Design review of the part built by this model. Coordinates are the model's own, in mm. Face numbers are marked on the shaded views. A direction names the side the tool comes from. Coordinates: 2 decimals unless noted, no trailing zeros. Loops run counter-clockwise (first coordinate to the right, second up) from the corner with the lowest first, then second, coordinate; pieces in that order, holes last. Notation, with made-up numbers: (-34.75, 20.25) - (-18.75, 20.25) arc R25 ccw to (-18.75, 53.25) - close; hole circle Ø1 at (12.5, 20). An arc over 180 degrees is marked (long way). Use one line per item in the form item = value. Start each with the question number.
(1) The part is to be moulded in two halves that separate along X. For the marked faces 3, 4, 5 and 6, say which applies: pulls with the +X half, pulls with the -X half, needs draft (parallel to the pull), parting line crosses it, or undercut.
(2) Add section D-D (x = 55.7). State the section outline as (y, z) points.
(3) For L1, parallel to X at y = 6.5, z = -1.35; L2, parallel to Y at x = 55.7, z = -3.3; L3, parallel to X at y = 19.5, z = -1.5, list the stretches that pass through material, from the lowest coordinate up.
(4) Add section C-C (y = 9.25). State the section outline as (x, z) points, plus the area to 3 significant figures.
(5) Tool access review of the marked faces 1 and 2: name each direction out of +Z, -Z, +X, -X, +Y, -Y from which nothing blocks a thin tool from reaching the whole face with its end or side.
(6) Add section A-A (y = -2). State the section outline as (x, z) points, plus the area to 3 significant figures.
(7) Clearance check with flat-ended pins moving along their axes: pin 1 Ø7.5 at (x, z) = (41, -9.5) entering from +Y; pin 2 Ø1.6 at (x, y) = (37, -1) entering from -Z. State where each tip first meets the part, or that it passes through.
(8) Add section B-B (x = 5.3). State the section outline as (y, z) points, plus the area to 3 significant figures.
Autodesk Inventor part; units mm, degrees
ref_plane "YZ Plane" through (0, 0, 0) normal (1, 0, 0) x (0, 1, 0)
ref_plane "XZ Plane" through (0, 0, 0) normal (0, 1, 0) x (-1, 0, 0)
ref_plane "XY Plane" through (0, 0, 0) normal (0, 0, 1) x (1, 0, 0)
sketch "Esquisse1" plane through (0, 0, 0) normal (0, 1, 0) x (-1, 0, 0)
  line L0 (0, 0) -> (-61, 0)
  line L1 (-61, 0) -> (-61, -15)
  line L2 (-61, -15) -> (0, -15)
  line L3 (0, -15) -> (0, 0)
  dimension "d0" = 15
  dimension "d1" = 61
extrude "Extrusion1" add sketch "Esquisse1" along normal blind 2
sketch "Esquisse2" plane through (0, 2, 0) normal (0, 1, 0) x (1, 0, 0)
  line L0 (0, 15) -> (0, 0)
  line L1 (0, 0) -> (9.5, 0)
  line L2 (9.5, 0) -> (9.5, 4.3)
  line L3 (0, 6.2) -> (0, 0)
  line L4 (0, 15) -> (9.5, 15)
  line L5 (9.5, 15) -> (9.5, 8.8)
  line L6 (9.5, 8.8) -> (0, 8.8)
  line L7 (0, 8.8) -> (0, 15)
  line L8 (0, 0) -> (61, 0) construction
  line L9 (30.5, 0) -> (30.5, 15) construction
  line L10 (61, 15) -> (61, 0)
  line L11 (61, 0) -> (51.5, 0)
  line L12 (51.5, 0) -> (51.5, 4.3)
  line L13 (51.5, 4.3) -> (61, 6.2)
  line L14 (61, 6.2) -> (61, 0)
  line L15 (61, 15) -> (51.5, 15)
  line L16 (51.5, 15) -> (51.5, 8.8)
  line L17 (51.5, 8.8) -> (61, 8.8)
  line L18 (61, 8.8) -> (61, 15)
  line L19 (0, 6.2) -> (2.5, 6.2)
  line L20 (2.5, 6.2) -> (9.5, 4.3)
  dimension "d33" = 2.6
  dimension "d34" = 6.2
  dimension "d36" = 4.5
  dimension "d37" = 2.5
  dimension "d38" = 7
extrude "Extrusion2" add sketch "Esquisse2" along normal blind 20
sketch "Esquisse3" plane through (0, 0, 0) normal (0, 0, 1) x (1, 0, 0)
  circle A0 centre (55.7, 16.5) radius 2
  line L0 (51.5, 2) -> (51.5, 22)
  circle A1 centre (55.7, 6.5) radius 2
  line L1 (51.5, 22) -> (61, 22)
  line L2 (0, 0) -> (61, 0)
  line L3 (51.5, 2) -> (9.5, 2) construction
  line L4 (30.5, 0) -> (30.5, 2) construction
  line L5 (9.5, 2) -> (51.5, 2) construction
  circle A2 centre (5.3, 16.5) radius 2
  circle A3 centre (5.3, 6.5) radius 2
  dimension "d10" = 4
  dimension "d11" = 4.2
  dimension "d12" = 4.2
  dimension "d40" = 10
  dimension "d41" = 4.5
extrude "Extrusion3" cut sketch "Esquisse3" against normal blind 20
sketch "Esquisse4" plane through (0, 0, 0) normal (0, -1, 0) x (1, 0, 0)
  circle A0 centre (44, -7.5) radius 5.15
  circle A1 centre (44, -7.5) radius 3.15
  line L0 (61, -6.2) -> (61, -8.8) construction
  line L1 (0, -8.8) -> (0, -6.2) construction
  line L2 (0, -15) -> (0, 0) construction
  line L3 (0, 0) -> (61, 0) construction
  line L4 (9.5, 0) -> (51.5, 0) construction
  line L5 (44, 0) -> (44, -15) construction
  line L6 (61, 0) -> (61, -15) construction
  line L7 (61, -15) -> (0, -15) construction
  dimension "d18" = 6.3
  dimension "d19" = 2
  dimension "d21" = 17
sketch "Esquisse5" plane through (0, 2, 0) normal (0, 1, 0) x (1, 0, 0)
  circle A0 centre (38, 7.5) radius 3.15
  line L0 (41.0311, 2.25) -> (34.9689, 2.25)
  line L1 (34.9689, 2.25) -> (31.9378, 7.5)
  line L2 (31.9378, 7.5) -> (34.9689, 12.75)
  line L3 (34.9689, 12.75) -> (41.0311, 12.75)
  line L4 (41.0311, 12.75) -> (44.0622, 7.5)
  line L5 (44.0622, 7.5) -> (41.0311, 2.25)
  line L6 (9.5, 0) -> (51.5, 0)
  point P0 (0, 0)
  dimension "d24" = 10.5
sketch "Esquisse7" plane through (0, 0, 0) normal (0, -1, 0) x (1, 0, 0)
  circle A0 centre (38, -7.5) radius 3.15
  circle A1 centre (38, -7.5) radius 7.5
  line L0 (61, -15) -> (0, -15)
  point P0 (0, 0)
extrude "Extrusion6" add sketch "Esquisse7" along normal blind 8
extrude "Extrusion7" cut sketch "Esquisse5" against normal blind 5.3 contours A0 | L0 L1 L2 L3 L4 L5
fillet "Congé1" radius 2 1 edges at (30.5, -8, -7.5)
equation "\"d12\" = d11"
properties part number "exp0"
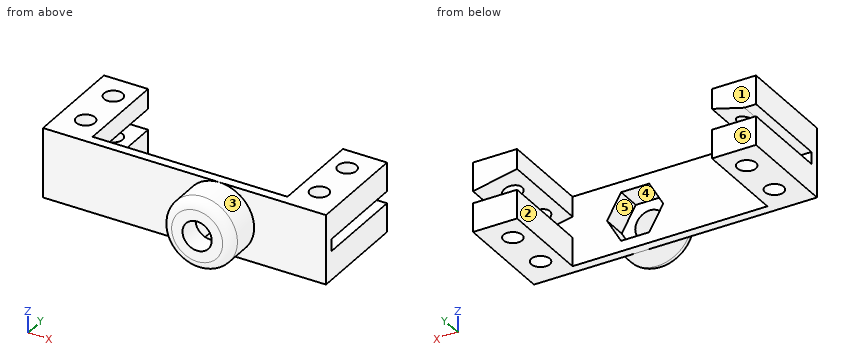
Computed values:
q1.face_3 = parting line crosses it
q1.face_4 = undercut
q1.face_5 = undercut
q1.face_6 = needs draft
q2.outline = (0, -15) - (4.5, -15) - (4.5, -8.8) - (2, -8.8) - (2, -5.14) - (4.5, -5.14) - (4.5, 0) - (0, 0) - close; (8.5, -15) - (14.5, -15) - (14.5, -8.8) - (8.5, -8.8) - close; (8.5, -5.14) - (14.5, -5.14) - (14.5, 0) - (8.5, 0) - close; (18.5, -15) - (22, -15) - (22, -8.8) - (18.5, -8.8) - close; (18.5, -5.14) - (22, -5.14) - (22, 0) - (18.5, 0) - close
q3.L1 = 0 to 3.3, 7.3 to 9.5, 51.5 to 53.7, 57.7 to 61
q3.L2 = 0 to 4.5, 8.5 to 14.5, 18.5 to 22
q3.L3 = 0 to 9.5, 51.5 to 61
q4.outline = (0, -15) - (9.5, -15) - (9.5, -8.8) - (0, -8.8) - close; (0, -6.2) - (2.5, -6.2) - (9.5, -4.3) - (9.5, 0) - (0, 0) - close; (51.5, -15) - (61, -15) - (61, -8.8) - (51.5, -8.8) - close; (51.5, -4.3) - (61, -6.2) - (61, 0) - (51.5, 0) - close
q4.area = 220 mm^2
q5.face_1 = +Z, -Z, +X, -X, +Y
q5.face_2 = +Z, -Z, +Y
q6.outline = circle Ø15 at (38, -7.5); hole (31.94, -7.5) - (34.97, -12.75) - (41.03, -12.75) - (44.06, -7.5) - (41.03, -2.25) - (34.97, -2.25) - close
q6.area = 81.2 mm^2
q7.pin_1 = 2
q7.pin_2 = -15
q8.outline = (0, -15) - (4.5, -15) - (4.5, -8.8) - (2, -8.8) - (2, -5.44) - (4.5, -5.44) - (4.5, 0) - (0, 0) - close; (8.5, -15) - (14.5, -15) - (14.5, -8.8) - (8.5, -8.8) - close; (8.5, -5.44) - (14.5, -5.44) - (14.5, 0) - (8.5, 0) - close; (18.5, -15) - (22, -15) - (22, -8.8) - (18.5, -8.8) - close; (18.5, -5.44) - (22, -5.44) - (22, 0) - (18.5, 0) - close
q8.area = 170 mm^2
